```python
from build123d import *

# Parameters (mm, degrees)
F0_R            = 45
F0_R_2          = 6.5
F1_DEPTH        = 3
F2_R            = 4.5
F3_DEPTH        = 25
F3_COPIES_COUNT = 6


# Not quite as in the source:
# - a pattern or mirror of a feature is missing from the dataset's text; its kind, count and spacing are read off the source's solid


with BuildPart() as f1:
    # F0 (on Front) → F1 (new body, symmetric)
    with BuildSketch(Plane.XZ):
        Circle(F0_R)
        Circle(F0_R_2, mode=Mode.SUBTRACT)
    extrude(amount=F1_DEPTH, both=True)

    # F2 (on face) → F3 (cut)
    with BuildSketch(Plane.XZ.offset(3)):
        with Locations((0, 37)):
            Circle(F2_R)
    f3 = extrude(amount=-F3_DEPTH, mode=Mode.SUBTRACT)

    # F3_copies: F3 ×6 about axis
    f3_copies_axis = Axis((0, 0, 0), (0, 1, 0))
    for i in range(1, F3_COPIES_COUNT):
        add(f3.rotate(f3_copies_axis, i * 360 / F3_COPIES_COUNT), mode=Mode.SUBTRACT)


solid = f1.part
```
Source: CAD feature listing. Evaluate the final solid. Frame: model axes, mm. Give positions to 0.01 mm unless a question says otherwise; leave off trailing zeros. Write each loop counter-clockwise with the first axis right and the second up, starting at its lowest first coordinate (ties: lowest second). Pieces come first, ordered by that corner, then holes.
1. Section query A-A (x = 0). Return the cut outline in (y, z), then the cut area to 3 significant figures.
2. First-contact query: pin 1 (1.5 mm diameter, centred on y = 0.5, z = -28, fed in from -X); pin 2 (3 mm diameter, centred on y = 0.5, z = 18, fed in from +X). Flat tips, straight axial feed; report the tip coordinate or a pass-through.
3. Section query D-D (y = -1.4). Return the cut outline in (x, z), then the cut area to 3 significant figures.
4. Pull-direction query (Z, two-part tool) for faces 1 (the face through (20.765, -0.042, -39.923)), 2 (the face through (0.98, -0.04, -32.61)), 3 (the face through (9, -3, 1)); classes: +Z half, -Z half, draft (parallel to the pull), parting line (faces both ways), or undercut.
5. Section query B-B (z = 0). Return the cut outline in (x, y), then the cut area to 3 significant figures.
6. Material intervals for line 1 along Z through (x, y) = (0, -0.05); line 2 along Z through (x, y) = (34, 1.6); line 3 along Z through (x, y) = (1.5, 0) (3 decimals), sorted ascending.
7. Section query C-C (z = 18.5). Return the cut outline in (x, y), then the cut area to 3 significant figures.
Output values:
1. outline: (-3, -45) - (3, -45) - (3, -41.5) - (-3, -41.5) - close; (-3, -32.5) - (3, -32.5) - (3, -6.5) - (-3, -6.5) - close; (-3, 6.5) - (3, 6.5) - (3, 32.5) - (-3, 32.5) - close; (-3, 41.5) - (3, 41.5) - (3, 45) - (-3, 45) - close
1. area: 354 mm2
2. pin 1: stops at x = -35.81
2. pin 2: stops at x = 41.87
3. outline: circle Ø90 at (0, 0); hole circle Ø9 at (-32.04, -18.5); hole circle Ø9 at (-32.04, 18.5); hole circle Ø13 at (0, 0); hole circle Ø9 at (0, -37); hole circle Ø9 at (0, 37); hole circle Ø9 at (32.04, -18.5); hole circle Ø9 at (32.04, 18.5)
3. area: 5,850 mm2
4. face 1: parting line
4. face 2: undercut
4. face 3: draft
5. outline: (-45, -3) - (-6.5, -3) - (-6.5, 3) - (-45, 3) - close; (6.5, -3) - (45, -3) - (45, 3) - (6.5, 3) - close
5. area: 462 mm2
6. line 1: z = -45 to -41.5, -32.5 to -6.5, 6.5 to 32.5, 41.5 to 45
6. line 2: z = -29.48 to -22.55, -14.45 to 14.45, 22.55 to 29.48
6. line 3: z = -44.975 to -41.243, -32.757 to -6.325, 6.325 to 32.757, 41.243 to 44.975
7. outline: (-41.02, -3) - (-36.54, -3) - (-36.54, 3) - (-41.02, 3) - close; (-27.54, -3) - (27.54, -3) - (27.54, 3) - (-27.54, 3) - close; (36.54, -3) - (41.02, -3) - (41.02, 3) - (36.54, 3) - close
7. area: 384 mm2
